Geometry check sheet. Reference: the model listing, model coordinates, mm. A direction names the side the tool comes from. Coordinates: 2 decimals unless noted, no trailing zeros. Loops run counter-clockwise (first coordinate to the right, second up) from the corner with the lowest first, then second, coordinate; pieces in that order, holes last. Notation, with made-up numbers: (50.25, -31) - (87.25, -31) arc R27 ccw to (87.25, -7) - close; hole circle Ø8 at (71, 2.5). An arc over 180 degrees is marked (long way). Write item = value, one per line. Start each with the question number.
from build123d import *
from build123d.topology import SkipClean

# Parameters (mm, degrees)
CUT_EXTRUDE_1_DEPTH      = 10.5
CUT_EXTRUDE_2_DEPTH      = 52.961524227
CUT_EXTRUDE_2_DEPTH_BACK = 52.961524227
EXTRUDE_1_REACH          = 40.678
SKETCH_4_R               = 5.75
CUT_EXTRUDE_3_DEPTH      = 52.961524227
CUT_EXTRUDE_3_DEPTH_BACK = 52.961524227
SKETCH_5_R               = 3.25
SKETCH_6_W               = 0.8
SKETCH_6_H               = 6
EXTRUDE_2_DEPTH          = 0.3
PATTERN_CIRCULAR_1_COUNT = 13


with BuildPart() as part:
    # Sketch 1 → Revolve 1 (revolve)
    with BuildSketch(Plane.XY, mode=Mode.PRIVATE) as revolve_1_sk:
        Polygon((36, 0), (0, 0), (0, -8.25), (6, -8.25), (6, -10), (20, -10), (20, -5.75), (36, -5.75), align=None)
    revolve(revolve_1_sk.sketch.rotate(Axis((0, 0, 0), (1, 0, 0)), 270), axis=Axis((0, 0, 0), (1, 0, 0)))

    # Sketch 2 → Cut-Extrude 1 (cut)
    with SkipClean():  # the faces are left unmerged after this step: merging them gives an invalid solid
        with BuildSketch(Plane(origin=(20, 0, 0), x_dir=(0, 0, -1), z_dir=(1, 0, 0))):
            with BuildLine():
                ThreePointArc((-4.979646072, 2.875), (-2.875, 4.979646072), (0, 5.75))
                Line((0, 5.75), (-2.299080153, 9.732123635))
                ThreePointArc((-2.299080153, 9.732123635), (-5, 8.660254038), (-7.278726225, 6.857123635))
                Line((-7.278726225, 6.857123635), (-4.979646072, 2.875))
            make_face()
            with BuildLine():
                ThreePointArc((4.979646072, 2.875), (5.554073501, 1.488209509), (5.75, 0))
                Line((5.75, 0), (10, 0))
                ThreePointArc((10, 0), (9.893888613, 1.452917105), (9.577806377, 2.875))
                Line((9.577806377, 2.875), (4.979646072, 2.875))
            make_face()
            with BuildLine():
                Line((-2.299080153, -9.732123635), (0, -5.75))
                ThreePointArc((0, -5.75), (-2.875, -4.979646072), (-4.979646072, -2.875))
                Line((-4.979646072, -2.875), (-7.278726225, -6.857123635))
                ThreePointArc((-7.278726225, -6.857123635), (-5, -8.660254038), (-2.299080153, -9.732123635))
            make_face()
        extrude(amount=-CUT_EXTRUDE_1_DEPTH, mode=Mode.SUBTRACT)


with BuildPart() as body_2:
    # Sketch 1_3 → Revolve 2 (revolve)
    with BuildSketch(Plane.XY, mode=Mode.PRIVATE) as revolve_2_sk:
        Polygon((50, 0), (36, 0), (36, -5.75), (36, -10), (50, -10), align=None)
    revolve(revolve_2_sk.sketch.rotate(Axis((0, 0, 0), (1, 0, 0)), 270), axis=Axis((0, 0, 0), (1, 0, 0)))

    # Sketch 3 → Cut-Extrude 2 (cut, two sides: drawn at the far end of the back side and taken through both)
    with BuildSketch(Plane.XY.offset(-CUT_EXTRUDE_2_DEPTH_BACK)):
        Polygon((36, -10), (36, 10), (46.25, 10), align=None)
    extrude(amount=CUT_EXTRUDE_2_DEPTH + CUT_EXTRUDE_2_DEPTH_BACK, mode=Mode.SUBTRACT)

    # Sketch 4 → Extrude 1 (add, up to next)
    with BuildSketch(Plane(origin=(36, 0, 0), x_dir=(0, 0, -1), z_dir=(1, 0, 0)), mode=Mode.PRIVATE) as extrude_1_sk1:
        with Locations(Location((0, 0, 0), (0, 0, 270))):
            Circle(SKETCH_4_R)
    extrude_1_tool1 = extrude(extrude_1_sk1.sketch, amount=EXTRUDE_1_REACH, mode=Mode.PRIVATE) - body_2.part

    add(part.part)  # Extrude 1 merges part
    add(extrude_1_tool1.solids().sort_by_distance((36, 0, 0))[0])

    # Sketch 5 → Cut-Extrude 3 (cut, two sides: drawn at the far end of the back side and taken through both)
    with BuildSketch(Plane(origin=(50, 0, 0), x_dir=(0, 0, -1), z_dir=(1, 0, 0)).offset(-CUT_EXTRUDE_3_DEPTH_BACK)):
        Circle(SKETCH_5_R)
    extrude(amount=CUT_EXTRUDE_3_DEPTH + CUT_EXTRUDE_3_DEPTH_BACK, mode=Mode.SUBTRACT)

    # Sketch 6 → Extrude 2 (add)
    with BuildSketch(Plane(origin=(50, 0, 0), x_dir=(0, 0, -1), z_dir=(1, 0, 0))):
        with Locations((0, 6.5)):
            Rectangle(SKETCH_6_W, SKETCH_6_H)
    extrude_2 = extrude(amount=EXTRUDE_2_DEPTH)

    # Pattern Circular 1: Extrude 2 ×13 about axis
    pattern_circular_1_axis = Axis((0, 0, 0), (1, 0, 0))
    for i in range(1, PATTERN_CIRCULAR_1_COUNT):
        add(extrude_2.rotate(pattern_circular_1_axis, i * 360 / PATTERN_CIRCULAR_1_COUNT))


solid = body_2.part
(1) Sectioned sample at C-C on x = 8. Enter the section's corners in (y, z).
(2) Sectioned sample at A-A on x = 21.5. Enter the section's corners in (y, z), plus the area to 3 significant figures.
(3) Scan lines: line 1 (Y direction, x = 24, z = 0); line 2 (Z direction, x = 44, y = 3); line 3 (X direction, y = -2.5, z = 5). Record each from-to range of solid material in increasing order.
(4) Tool access check on faces 1 (the face through (9.5, 6, 4)), 2 (the face through (6, -7.5, 3.8)), 3 (the face through (50.3, -2.3, 6.1)). Record the directions out of +Z, -Z, +X, -X, +Y, -Y that give a thin tool (end or side, any length) a straight path to the whole face; none if there is none.
(5) Depth check by flat-ended pin: pin 1 (10 mm diameter, centred on y = 1.5, z = -3.5, fed in from +X); pin 2 (6 mm diameter, centred on x = 29, y = 7.5, fed in from +Z); pin 3 (2 mm diameter, centred on y = -8, z = 5, fed in from +X); pin 4 (1 mm diameter, centred on x = 16, y = -2, fed in from -Z). Enter the tip coordinate at first touch or a pass-through.
(6) Sectioned sample at B-B on x = 43. Enter the section's corners in (y, z), plus the area to 3 significant figures.
(7) Draft check along Y on faces 4 (the face through (44.654, -9.915, -1.302)), 5 (the face through (9.5, 1, -7)), 6 (the face through (20, 0, 7)). Enter one of: pulls with the +Y half, pulls with the -Y half, needs draft (parallel to the pull), parting line crosses it, or undercut.
Working result:
q1.outline = circle Ø20 at (0, 0); hole circle Ø6.5 at (0, 0)
q2.outline = circle Ø11.5 at (0, 0); hole circle Ø6.5 at (0, 0)
q2.area = 70.7 mm2
q3.line_1 = -5.75 to -3.25, 3.25 to 5.75
q3.line_2 = -9.54 to -1.25, 1.25 to 9.54
q3.line_3 = 0 to 50
q4.face_1 = none
q4.face_2 = -X
q4.face_3 = +Z, -Z, +X, +Y, -Y
q5.pin_1 = 50.3
q5.pin_2 = 3.58
q5.pin_3 = 50
q5.pin_4 = -9.89
q6.outline = (3.66, -9.31) - (3.66, -4.44) arc R5.75 ccw to (3.66, 4.44) - (3.66, 9.31) arc R10 ccw (long way) to start; hole circle Ø6.5 at (0, 0)
q6.area = 208 mm2
q7.face_4 = parting line crosses it
q7.face_5 = undercut
q7.face_6 = needs draft
